from build123d import *

# Parameters (mm, degrees)
SKETCH_1_W             = 6.25
SKETCH_1_H             = 5.1
EXTRUDE_1_DEPTH        = 13.3
SKETCH_2_W             = 6.25
SKETCH_2_H             = 8.86
CUT_EXTRUDE_1_DEPTH    = 3
SKETCH_7_W             = 12.5
SKETCH_7_H             = 8.86
CUT_EXTRUDE_2_DEPTH    = 1
SKETCH_8_W             = 12.5
SKETCH_8_H             = 1.005646511
EXTRUDE_2_DEPTH        = 0.5
SKETCH_9_W             = 1
SKETCH_9_H             = 1.1
CUT_EXTRUDE_3_DEPTH    = 8.86
SKETCH_6_W             = 0.4
SKETCH_6_H             = 0.4
PATTERN_LINEAR_1_COUNT = 4
PATTERN_LINEAR_1_PITCH = 2.6
SKETCH_10_W            = 10.5
SKETCH_10_H            = 3
CUT_EXTRUDE_4_DEPTH    = 2


with BuildPart() as part:
    # Эскиз1 → Бобышка-Вытянуть1 (new body)
    with BuildSketch(Plane.XY):
        with Locations((-3.125, 2.55)):
            Rectangle(SKETCH_1_W, SKETCH_1_H)
    extrude(amount=-EXTRUDE_1_DEPTH)

    # Эскиз2 → Вырез-Вытянуть1 (cut)
    with BuildSketch(Plane.XZ):
        with Locations((-3.125, -4.43)):
            Rectangle(SKETCH_2_W, SKETCH_2_H)
    extrude(amount=-CUT_EXTRUDE_1_DEPTH, mode=Mode.SUBTRACT)

    # Зеркальное отражение1: part across plane


with BuildPart() as part_1:
    add(part.part)
    add(part.part.mirror(Plane(origin=(0, 5.1, -13.3), x_dir=(0, 0, 1), z_dir=(1, 0, 0))))

    # Эскиз7 → Вырез-Вытянуть2 (cut)
    with BuildSketch(Plane(origin=(0, 5.1, 0), x_dir=(1, 0, 0), z_dir=(0, 1, 0))):
        with Locations((0, 4.43)):
            Rectangle(SKETCH_7_W, SKETCH_7_H)
    extrude(amount=-CUT_EXTRUDE_2_DEPTH, mode=Mode.SUBTRACT)

    # Эскиз8 → Бобышка-Вытянуть2 (add)
    with BuildSketch(Plane(origin=(0, 0, 0), x_dir=(-1, 0, 0), z_dir=(0, -1, 0))):
        with Locations((0, 9.362823256)):
            Rectangle(SKETCH_8_W, SKETCH_8_H)
    extrude(amount=EXTRUDE_2_DEPTH)

    # Эскиз9 → Вырез-Вытянуть3 (cut)
    with BuildSketch(Plane.XY):
        with Locations((5.75, 3.55)):
            Rectangle(SKETCH_9_W, SKETCH_9_H)
        with Locations((-5.75, 3.55)):
            Rectangle(SKETCH_9_W, SKETCH_9_H)
    extrude(amount=-CUT_EXTRUDE_3_DEPTH, mode=Mode.SUBTRACT)

    # Вырез-По траектории1: sweep along a curve in space
    with BuildLine() as sweep_1_path:
        Line((-3.88435792, 3, 0), (-3.88435792, 3, -13.1))
        Line((-3.88435792, 3, -13.1), (-3.88435792, -0.439783166, -13.1))
    # Эскиз6 → Вырез-По траектории1 (sweep, cut)
    with BuildSketch(Plane.XY):
        with Locations((-3.88435792, 3)):
            Rectangle(SKETCH_6_W, SKETCH_6_H)
    sweep_1 = sweep(path=sweep_1_path.line, transition=Transition.RIGHT, mode=Mode.SUBTRACT)

    # Линейный массив1: Вырез-По траектории1 ×4
    with Locations(*[(i * PATTERN_LINEAR_1_PITCH, 0, 0) for i in range(1, PATTERN_LINEAR_1_COUNT)]):
        add(sweep_1, mode=Mode.SUBTRACT)

    # Эскиз10 → Вырез-Вытянуть4 (cut)
    with BuildSketch(Plane(origin=(0, 0, -13.3), x_dir=(-1, 0, 0), z_dir=(0, 0, -1))):
        with Locations((0, 3.6)):
            Rectangle(SKETCH_10_W, SKETCH_10_H)
    extrude(amount=-CUT_EXTRUDE_4_DEPTH, mode=Mode.SUBTRACT)


solid = part_1.part
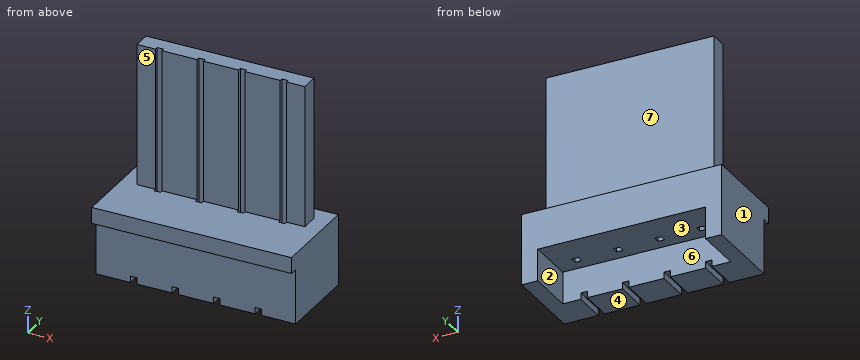
Read the model definition and answer for the solid it produces. Units are mm, in the model's axes. Face numbers are marked on the shaded views. A direction names the side the tool comes from. Give positions to 0.01 mm unless a question says otherwise; leave off trailing zeros. Write each loop counter-clockwise with the first axis right and the second up, starting at its lowest first coordinate (ties: lowest second). Pieces come first, ordered by that corner, then holes. Notation, with made-up numbers: (88, -33) - (128, -33) arc R16 cw to (128, -23) - close; hole circle Ø11 at (7.25, 51). An arc over 180 degrees is marked (long way). Answer in a Markdown table with one row per item. Add a question column.
Item 1: Flat-ended cylindrical pins translate along their axes: P1, Ø2.5, axis at x = 0, z = -3.5, coming from the -Y side; P2, Ø5, axis at x = 1.5, z = -12, coming from the +Y side; P3, Ø3, axis at x = -1, z = -4, coming from the +Y side. Find the tip coordinate at first contact, or state that the pin passes through.
Item 2: A tool of negligible diameter and unlimited length cuts with its end or side. For the marked faces 5, 6 and 7, from which of +Z, -Z, +X, -X, +Y, -Y can it reach the whole face along a straight path? Write none if from no direction.
Item 3: Section A-A, the plane x = 0.5 is taken. Write down the section's boundary in (y, z), and give its area (3 significant figures).
Item 4: Section C-C, the plane z = -7.5 is taken. Write down the section's boundary in (x, y), and give its area (3 significant figures).
Item 5: Section D-D, the plane y = 4.5 is taken. Write down the section's boundary in (x, z).
Item 6: Section B-B, the plane y = 3.7 is taken. Write down the section's boundary in (x, z).
Item 7: Find the intervals of material crossed by L1, parallel to Y at x = 4, z = -10; L2, parallel to X at y = 3.1, z = -12.5; L3, parallel to Z at x = -4.25, y = 1, in increasing order.
Item 8: Determine the mould class of the marked faces 1, 2, 3 and 4 for opening direction X: pulls with the +X half, pulls with the -X half, needs draft (parallel to the pull), parting line crosses it, or undercut.
Recorded:
| question | item | result |
|---|---|---|
| 1 | P1 | stops at y = 3 |
| 1 | P2 | stops at y = 5.1 |
| 1 | P3 | stops at y = 4.1 |
| 2 | face 5 | +Z, +X, -X, -Y |
| 2 | face 6 | -Z, +Y |
| 2 | face 7 | +Z, +X, -X, +Y |
| 3 | outline | (-0.5, -9.87) - (0, -9.87) - (0, -13.3) - (2.1, -13.3) - (2.1, -11.3) - (5.1, -11.3) - (5.1, -8.86) - (4.1, -8.86) - (4.1, 0) - (3, 0) - (3, -8.86) - (-0.5, -8.86) - close |
| 3 | area | 26.9 mm2 |
| 4 | outline | (-5.25, 3) - (-4.08, 3) - (-4.08, 3.2) - (-3.68, 3.2) - (-3.68, 3) - (-1.48, 3) - (-1.48, 3.2) - (-1.08, 3.2) - (-1.08, 3) - (1.12, 3) - (1.12, 3.2) - (1.52, 3.2) - (1.52, 3) - (3.72, 3) - (3.72, 3.2) - (4.12, 3.2) - (4.12, 3) - (5.25, 3) - (5.25, 4.1) - (-5.25, 4.1) - close |
| 4 | area | 11.2 mm2 |
| 5 | outline | (-6.25, -13.3) - (-5.25, -13.3) - (-5.25, -11.3) - (5.25, -11.3) - (5.25, -13.3) - (6.25, -13.3) - (6.25, -8.86) - (-6.25, -8.86) - close |
| 6 | outline | (-6.25, -13.3) - (-5.25, -13.3) - (-5.25, -11.3) - (5.25, -11.3) - (5.25, -13.3) - (6.25, -13.3) - (6.25, -8.86) - (5.25, -8.86) - (5.25, 0) - (-5.25, 0) - (-5.25, -8.86) - (-6.25, -8.86) - close |
| 7 | L1 | y = 0 to 2.8, 3.2 to 5.1 |
| 7 | L2 | x = -6.25 to -5.25, 5.25 to 6.25 |
| 7 | L3 | z = -13.3 to -8.86 |
| 8 | face 1 | pulls with the -X half |
| 8 | face 2 | undercut |
| 8 | face 3 | undercut |
| 8 | face 4 | needs draft |
